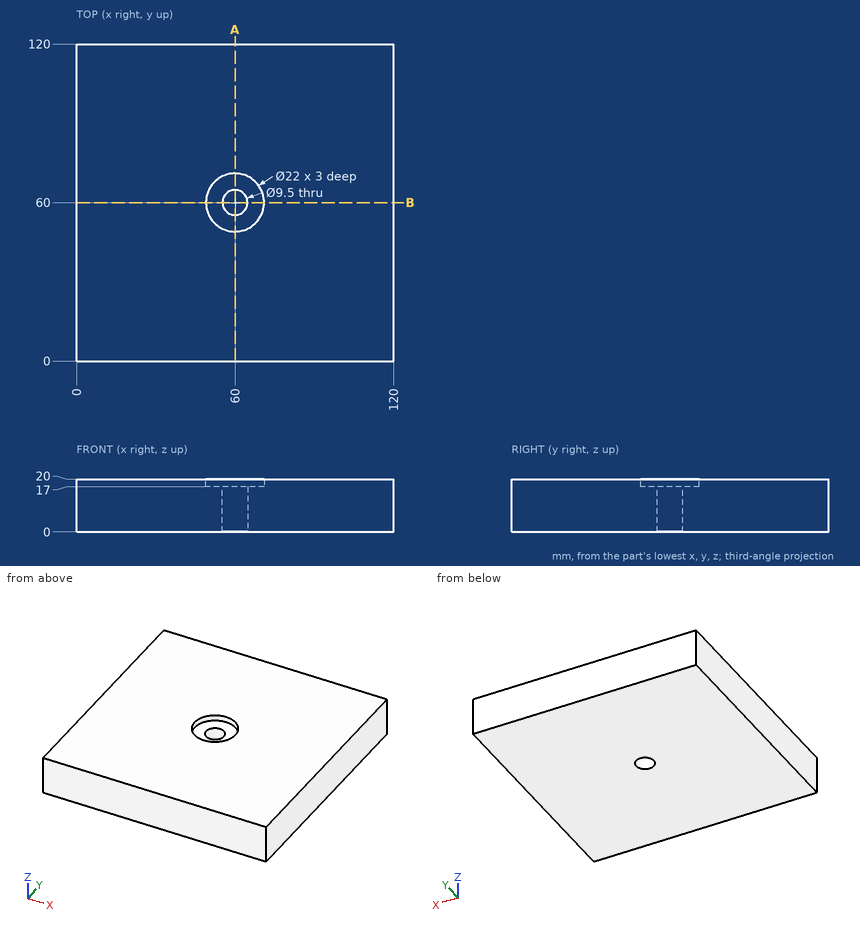
The figure shows three views and two pictorial views of one solid part (mm, origin at its lowest corner). Answer the questions. Give positions to 0.01 mm unless a question says otherwise; leave off trailing zeros. Write each loop counter-clockwise with the first axis right and the second up, starting at its lowest first coordinate (ties: lowest second). Pieces come first, ordered by that corner, then holes. Notation, with made-up numbers: (82.5, 81.25) -> (87.5, 81.25) arc R26 ccw to (87.5, 114.25) -> close; hole circle Ø2 at (-35.75, -24.5). An arc over 180 degrees is marked (long way). Answer as a JSON object with one key per item and string values.
1) Straight lines are drawn through the part: probe 1 along Y at (x, z) = (60, 8.5); probe 2 along Y at (x, z) = (60, 19.35). For each, find the intervals that lie inside material, in ascending order. Write a range as from..to.
Findings below:
{"probe 1": "y = 0..55.25, 64.75..120", "probe 2": "y = 0..49, 71..120"}
2) Section A-A on x = 60 is taken. Write down the section's boundary in (y, z), then the cut area to 3 significant figures.
Findings below:
{"outline": "(0, 0) -> (55.25, 0) -> (55.25, 17) -> (49, 17) -> (49, 20) -> (0, 20) -> close; (64.75, 0) -> (120, 0) -> (120, 20) -> (71, 20) -> (71, 17) -> (64.75, 17) -> close", "area": "2,170 mm^2"}
3) Flat-ended cylindrical pins translate along their axes: pin 1 Ø13 at (x, y) = (60, 60) entering from -Z; pin 2 Ø5.5 at (x, y) = (60, 60) entering from +Z. Find the tip coordinate at first contact, or state that the pin passes through.
Findings below:
{"pin 1": "stops at z = 0", "pin 2": "passes through"}
